Geometry check sheet. Reference: the model listing, model coordinates, mm. A direction names the side the tool comes from. Round coordinates to 2 decimals unless told otherwise and drop trailing zeros. Order: outer loops, then holes, each group sorted by start corner. A loop starts at its lowest first (then second) coordinate and runs counter-clockwise, first axis right, second up. Notation, with made-up numbers: (-36, 27) -> (8, 27) arc R34 ccw to (8, 60) -> close; hole circle Ø9 at (51.25, 86). An arc over 180 degrees is marked (long way). Use a Markdown table: item, result. Add a question column.
Item 1: Mould release check, pull along Y, two halves, no side actions. Record for faces 5 (the cylindrical face through (-26.42, -5.46, 0.36)), 6 (the flat face through (-11.204, -22.016, 7.43)), 7 (the flat face through (-8.17, 19.64, 7.43)): pulls with the +Y half, pulls with the -Y half, needs draft (parallel to the pull), parting line crosses it, or undercut.
Item 2: Set-up check for faces 1 (the flat face through (-11.27, -21.94, -7.5)), 2 (the flat face through (31.53, 6.92, 3.99)), 3 (the flat face through (34, 14, 5)), 4 (the flat face through (-12, 24, 1.5)): record each of +Z, -Z, +X, -X, +Y, -Y from which the full face is reachable in a straight line by a thin tool's end or side.
Item 3: Gauge pin test, flat ends, axial feed: pin 1 Ø3 at (x, y) = (-11, 23) entering from +Z; pin 2 Ø6.5 at (x, y) = (-10, 29) entering from +Z; pin 3 Ø5 at (x, y) = (24.27, 6.31) entering from -Z. Record the tip position at first contact, or that the pin passes through.
Item 4: Sectioned sample at A-A, the plane z = -7.5. Record the cut outline in (x, y), and give its area (3 significant figures).
Item 5: Material ranges on probe 1 along Z at (x, y) = (0.5, -1); probe 2 along Y at (x, z) = (-30.5, -7.25); probe 3 along Y at (x, z) = (-29, -4.5), recorded low to high. Write a range as [from, to].
Item 6: Sectioned sample at B-B, the plane x = 29.5. State how many separate pieces and enclosed holes the cut face has, and give its area (3 significant figures).
from build123d import *

# Parameters (mm, degrees)
BOSS_EXTRU_1_DEPTH      = 80
BOSS_EXTRU_2_DEPTH      = 80
ESQUISSE6_R             = 10
ENL_V_MAT_EXTRU_1_DEPTH = 94.48690022224822
ESQUISSE7_R             = 10.000000000000004
ENL_V_MAT_EXTRU_2_DEPTH = 94.48690022224821
ENL_V_START             = -2
ESQUISSE8_R             = 2.9999999999999973
ESQUISSE8_R_2           = 3.0000000000000004
ENL_V_MAT_EXTRU_3_DEPTH = 10


with BuildPart() as part:
    # Esquisse4 → Boss.-Extru.1 (new body)
    with BuildSketch(Plane(origin=(31.486834784070687, 24.669398762041954, 0), x_dir=(0, 0, 1), z_dir=(-0.7871708696017671, -0.6167349690510487, 0))):
        with BuildLine():
            Line((-9.92847971530262, -6.739828673106199), (-5.000000000000012, -13.999999999999998))
            Line((-5.000000000000012, -13.999999999999998), (1.4999999999999891, -14.000000000000004))
            Line((1.4999999999999891, -14.000000000000004), (1.4999999999999891, -9.886859966642595))
            ThreePointArc((1.4999999999999891, -9.886859966642595), (-2.2566974751833473, 9.742038621638756), (2.9999999999999933, -9.539392014169461))
            Line((2.9999999999999933, -9.539392014169461), (2.999999999999988, -14.000000000000005))
            Line((2.999999999999988, -14.000000000000005), (4.999999999999987, -14.000000000000009))
            Line((4.999999999999987, -14.000000000000009), (9.928479715302606, -6.739828673106216))
            ThreePointArc((9.928479715302606, -6.739828673106216), (1.807e-14, 12), (-9.92847971530262, -6.739828673106199))
        make_face()
    extrude(amount=BOSS_EXTRU_1_DEPTH)

    # Esquisse5 → Boss.-Extru.2 (add)
    with BuildSketch(Plane(origin=(31.48683478407068, -24.66939876204195, 0), x_dir=(0, 0, -1), z_dir=(0.7871708696017671, -0.6167349690510487, 0))):
        with BuildLine():
            Line((9.9284797153026, 6.7398286731062225), (4.999999999999976, 14.000000000000009))
            Line((4.999999999999976, 14.000000000000009), (-1.5000000000000255, 13.999999999999995))
            Line((-1.5000000000000255, 13.999999999999995), (-1.5000000000000149, 9.88685996664259))
            ThreePointArc((-1.5000000000000149, 9.88685996664259), (2.256697475183369, -9.742038621638747), (-3.0000000000000173, 9.53939201416945))
            Line((-3.0000000000000173, 9.53939201416945), (-3.0000000000000244, 13.999999999999996))
            Line((-3.0000000000000244, 13.999999999999996), (-5.000000000000023, 13.999999999999991))
            Line((-5.000000000000023, 13.999999999999991), (-9.928479715302622, 6.739828673106189))
            ThreePointArc((-9.928479715302622, 6.739828673106189), (1.777e-14, -11.999999999999998), (9.9284797153026, 6.7398286731062225))
        make_face()
    extrude(amount=-BOSS_EXTRU_2_DEPTH)

    # Esquisse6 → Enlèv. mat.-Extru.1 (cut, through all)
    with BuildSketch(Plane(origin=(31.486834784070695, 24.669398762041958, 0), x_dir=(0, 0, -1), z_dir=(0.7871708696017669, 0.6167349690510489, 0))):
        with Locations(Location((0, 6.94e-15, 0), (0, 0, 252.542396876))):
            Circle(ESQUISSE6_R)
    extrude(amount=-ENL_V_MAT_EXTRU_1_DEPTH, mode=Mode.SUBTRACT)

    # Esquisse7 → Enlèv. mat.-Extru.2 (cut, through all)
    with BuildSketch(Plane(origin=(31.486834784070687, -24.669398762041954, 0), x_dir=(0, 0, -1), z_dir=(0.7871708696017669, -0.6167349690510489, 0))):
        with Locations(Location((0, -6.94e-15, 0), (0, 0, 98.626926559))):
            Circle(ESQUISSE7_R)
    extrude(amount=-ENL_V_MAT_EXTRU_2_DEPTH, mode=Mode.SUBTRACT)

    # Esquisse8 → Enlèv. mat.-Extru.3 (cut)
    with BuildSketch(Plane(origin=(5e-17, -5.97e-15, 2.999999999999953), x_dir=(-1, 0, 2e-17), z_dir=(-2e-17, 1.99e-15, -1)).offset(ENL_V_START)):
        with Locations(Location((21.383630745551354, 29.45743261280437, 0), (0, 0, 128.078094677))):
            Circle(ESQUISSE8_R)
        with Locations(Location((11.937580310330151, 22.056612984191787, 0), (0, 0, 128.078094677))):
            Circle(ESQUISSE8_R_2)
        with Locations(Location((-24.272279691351134, 6.31319559215644, 0), (0, 0, 115.397306959))):
            Circle(ESQUISSE8_R)
        with Locations(Location((-33.71833012657233, 13.714015220769031, 0), (0, 0, 115.397306959))):
            Circle(ESQUISSE8_R_2)
    extrude(amount=-ENL_V_MAT_EXTRU_3_DEPTH, mode=Mode.SUBTRACT)


solid = part.part
Found:
| question | item | result |
|---|---|---|
| 1 | face 5 | undercut |
| 1 | face 6 | pulls with the -Y half |
| 1 | face 7 | pulls with the +Y half |
| 2 | face 1 | -Z, -Y |
| 2 | face 2 | +Z, -Z, +X |
| 2 | face 3 | +Z |
| 2 | face 4 | +Y |
| 3 | pin 1 | stops at z = 5 |
| 3 | pin 2 | stops at z = 5.4 |
| 3 | pin 3 | stops at z = -9.41 |
| 4 | outline | (-37.26, -17.3) -> (-35.57, -19.46) -> (-10.72, 0) -> (-35.57, 19.46) -> (-37.26, 17.3) -> (-15.19, 0) -> close; (-27.41, -29.88) -> (-25.12, -32.79) -> (0.77, -12.5) -> (25.71, -32.04) -> (27.41, -29.88) -> (0, -8.4) -> close; (-27.41, 29.88) -> (0, 8.4) -> (27.41, 29.88) -> (25.71, 32.04) -> (0.77, 12.5) -> (-25.12, 32.79) -> close; (10.72, 0) -> (35.57, -19.46) -> (37.85, -16.55) -> (16.73, 0) -> (37.85, 16.55) -> (35.57, 19.46) -> close |
| 4 | area | 814 mm2 |
| 5 | probe 1 | z = [-11.99, -9.99], [9.99, 11.99] |
| 5 | probe 2 | y = [-15.15, -11.75], [11.75, 15.15] |
| 5 | probe 3 | y = [-11.38, -8.59], [8.59, 11.38] |
| 6 | separate pieces | 4 |
| 6 | enclosed holes | 0 |
| 6 | area | 281 mm2 |
